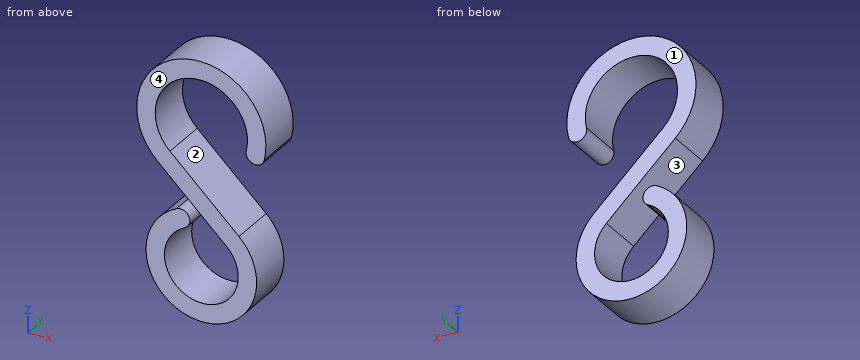
from build123d import *

# Parameters (mm, degrees)
F1_DEPTH = 12.5


with BuildPart() as f1:
    # F0 (on Front) → F1 (new body)
    with BuildSketch(Plane.XZ):
        with BuildLine():
            ThreePointArc((-8.63434, -9.313333), (-3.748413, 12.134224), (12.382753, -2.820891))
            ThreePointArc((12.382753, -2.820891), (14.295126, -5.86162), (17.335854, -3.949247))
            ThreePointArc((17.335854, -3.949247), (-5.247779, 16.987914), (-12.088076, -13.038667))
            Line((-12.088076, -13.038667), (6.907472, -30.649333))
            ThreePointArc((6.907472, -30.649333), (-1.427534, -48.159212), (-4.561795, -29.021695))
            ThreePointArc((-4.561795, -29.021695), (-3.432667, -25.61167), (-6.842692, -24.482542))
            ThreePointArc((-6.842692, -24.482542), (-2.1413, -53.188818), (10.361208, -26.924))
            Line((10.361208, -26.924), (-8.63434, -9.313333))
        make_face()
    extrude(amount=F1_DEPTH)


solid = f1.part
Work out the finished part from the listing and answer in its coordinate system (mm). Face numbers are marked on the shaded views. A direction names the side the tool comes from. Coordinates: 2 decimals unless noted, no trailing zeros. Loops run counter-clockwise (first coordinate to the right, second up) from the corner with the lowest first, then second, coordinate; pieces in that order, holes last. Notation, with made-up numbers: M 24,6 L 54,6 A9 cw 54,20 Z; hole C -21,-17 d3. An arc over 180 degrees is marked long. Answer in a Markdown table with one row per item. Add a question column.
1. Consider L1, parallel to Z at x = 0, y = -7.5; L2, parallel to Z at x = -4.5, y = -3.5; L3, parallel to Z at x = 9, y = -3.25. Determine where each line is inside the solid, lowest interval first.
2. Find section A-A, the plane x = 4. Write down the section's boundary in (y, z).
3. The mould has two halves that part along Z. Classify the marked faces 1 and 2: pulls with the +Z half, pulls with the -Z half, needs draft (parallel to the pull), parting line crosses it, or undercut.
4. Flat-ended cylindrical pins translate along their axes: P1, Ø3, axis at x = 11, z = -0.5, coming from the -Y side; P2, Ø3, axis at y = -7, z = 7.5, coming from the +X side; P3, Ø4, axis at x = -7, y = -10, coming from the +Z side; P4, Ø1, axis at y = -5.5, z = -31.5, coming from the +X side. Find the tip coordinate at first contact, or state that the pin passes through.
5. Find section D-D, the plane x = 0. Write down the section's boundary in (y, z).
6. A tool of negligible diameter and unlimited length cuts with its end or side. For the marked faces 3 and 4, from which of +Z, -Z, +X, -X, +Y, -Y can it reach the whole face along a straight path? Write none if from no direction.
7. Find section C-C, the plane y = -8.5. Write down the section's boundary in (x, z), then the cut area to 3 significant figures.
8. Find section B-B, the plane z = 0. Write down the section's boundary in (x, y), then the cut area to 3 significant figures.
Reported:
| question | item | result |
|---|---|---|
| 1 | L1 | z = -53.34 to -48.26, -24.25 to -17.32, 12.7 to 17.78 |
| 1 | L2 | z = -52.66 to -47.21, -28.99 to -24.51, -20.07 to -13.15, 11.88 to 17.2 |
| 1 | L3 | z = -50.4 to -42.81, -33.39 to -25.66, 8.96 to 15.33 |
| 2 | outline | M -12.5,-52.81 L 0,-52.81 L 0,-47.44 L -12.5,-47.44 Z; M -12.5,-27.95 L 0,-27.95 L 0,-21.03 L -12.5,-21.03 Z; M -12.5,12.05 L 0,12.05 L 0,17.32 L -12.5,17.32 Z |
| 3 | face 1 | needs draft |
| 3 | face 2 | undercut |
| 4 | P1 | passes through |
| 4 | P2 | stops at x = 16.74 |
| 4 | P3 | stops at z = 17.06 |
| 4 | P4 | stops at x = 13.97 |
| 5 | outline | M -12.5,-53.34 L 0,-53.34 L 0,-48.26 L -12.5,-48.26 Z; M -12.5,-24.25 L 0,-24.25 L 0,-17.32 L -12.5,-17.32 Z; M -12.5,12.7 L 0,12.7 L 0,17.78 L -12.5,17.78 Z |
| 6 | face 3 | +Y, -Y |
| 6 | face 4 | +Z, -Z, +X, -X, -Y |
| 7 | outline | M -12.09,-13.04 L 6.91,-30.65 A10.16 cw long -4.56,-29.02 A2.54 ccw -6.84,-24.48 A15.24 ccw long 10.36,-26.92 L -8.63,-9.31 A12.7 cw long 12.38,-2.82 A2.54 ccw 17.34,-3.95 A17.78 ccw long Z |
| 7 | area | 803 mm^2 |
| 8 | outline | M -17.78,-12.5 L -12.7,-12.5 L -12.7,0 L -17.78,0 Z; M 12.7,-12.5 L 17.78,-12.5 L 17.78,0 L 12.7,0 Z |
| 8 | area | 127 mm^2 |
